Input: part model. Units: mm. Frame: model coordinates. A direction names the side the tool comes from. Coordinates: 2 decimals unless noted, no trailing zeros. Loops run counter-clockwise (first coordinate to the right, second up) from the corner with the lowest first, then second, coordinate; pieces in that order, holes last.
```python
from build123d import *

# Parameters (mm, degrees)
SKETCH1_W                                           = 68.2625
SKETCH1_H                                           = 190.5
BOSS_EXTRUDE1_DEPTH                                 = 20
CHAMFER1_SIZE                                       = 4
M8_TAPPED_HOLE1_D                                   = 6.8
F_8_0_8_DIAMETER_HOLE1_D                            = 8
CUT_EXTRUDE1_DEPTH                                  = 11
FILLET1_R                                           = 0.254
CBORE_FOR_M6_HEX_SOCKET_HEAD_CAP_SCREW1_D           = 6.6
CBORE_FOR_M6_HEX_SOCKET_HEAD_CAP_SCREW1_CBORE_D     = 11
CBORE_FOR_M6_HEX_SOCKET_HEAD_CAP_SCREW1_CBORE_DEPTH = 7
M6_TAPPED_HOLE1_D                                   = 5
M6_TAPPED_HOLE1_DEPTH                               = 27.9908
M6_TAPPED_HOLE1_TIP                                 = 1.502151548


with BuildPart() as part:
    # Sketch1 → Boss-Extrude1 (new body)
    with BuildSketch(Plane(origin=(0, 0, 0), x_dir=(1, 0, 0), z_dir=(0, 1, 0))):
        with Locations((-34.13125, 0)):
            Rectangle(SKETCH1_W, SKETCH1_H)
    extrude(amount=BOSS_EXTRUDE1_DEPTH)

    # Chamfer1
    chamfer1_edges = [part.edges().sort_by_distance(p)[0] for p in [
        (-34.13125, 20, -95.25),
    ]]
    chamfer(chamfer1_edges, length=CHAMFER1_SIZE)

    # M8 Tapped Hole1 (through all)
    with Locations(Plane(origin=(0, 20, 0), x_dir=(1, 0, 0), z_dir=(0, 1, 0))):
        with Locations((-59.85, -62.25), (-54.1, -32.25), (-19.1, -32.25), (-59.85, 37.75), (-54.1, 67.75), (-19.1, 67.75)):
            Hole(M8_TAPPED_HOLE1_D / 2)

    # Ø8.0 (8) Diameter Hole1 (through all)
    with Locations(Plane(origin=(0, 20, 0), x_dir=(1, 0, 0), z_dir=(0, 1, 0))):
        with Locations((-59.85, 20.0208), (-59.85, -79.9792)):
            Hole(F_8_0_8_DIAMETER_HOLE1_D / 2)

    # Sketch6 → Cut-Extrude1 (cut)
    with BuildSketch(Plane.XZ):
        with BuildLine():
            Line((-68.2625, 85.1242), (-54.85, 85.1242))
            ThreePointArc((-54.85, 85.1242), (-49.705, 79.9792), (-54.85, 74.8342))
            Line((-54.85, 74.8342), (-68.2625, 74.8342))
            ThreePointArc((-68.2625, 74.8342), (-73.4075, 79.9792), (-68.2625, 85.1242))
        make_face()
        with BuildLine():
            Line((-68.2625, -14.8758), (-54.85, -14.8758))
            ThreePointArc((-54.85, -14.8758), (-49.705, -20.0208), (-54.85, -25.1658))
            Line((-54.85, -25.1658), (-68.2625, -25.1658))
            ThreePointArc((-68.2625, -25.1658), (-73.4075, -20.0208), (-68.2625, -14.8758))
        make_face()
    extrude(amount=-CUT_EXTRUDE1_DEPTH, mode=Mode.SUBTRACT)

    # Fillet1
    fillet1_edges = [part.edges().sort_by_distance(p)[0] for p in [
        (-61.55625, 11, 85.1242),
        (-49.705, 11, 79.9792),
        (-61.55625, 11, 74.8342),
        (-61.55625, 11, -14.8758),
        (-49.705, 11, -20.0208),
        (-61.55625, 11, -25.1658),
    ]]
    fillet(fillet1_edges, radius=FILLET1_R)

    # CBORE for M6 Hex Socket Head Cap Screw1 (through all)
    with Locations(Plane(origin=(0, 0, 0), x_dir=(-1, 0, 0), z_dir=(0, -1, 0))):
        with Locations((9.849999954, 86.434800002), (39.849999954, 86.434800002), (39.849999954, -13.565199998), (9.849999954, -13.565199998)):
            CounterBoreHole(CBORE_FOR_M6_HEX_SOCKET_HEAD_CAP_SCREW1_D / 2, CBORE_FOR_M6_HEX_SOCKET_HEAD_CAP_SCREW1_CBORE_D / 2, CBORE_FOR_M6_HEX_SOCKET_HEAD_CAP_SCREW1_CBORE_DEPTH)

    # M6 Tapped Hole1
    with Locations(Plane(origin=(0, 0, 0), x_dir=(-1, 0, 0), z_dir=(0, -1, 0))):
        with Locations((42.35, 21.249999996), (42.35, 53.249999996)):
            Hole(M6_TAPPED_HOLE1_D / 2, depth=M6_TAPPED_HOLE1_DEPTH)
            with Locations((0, 0, -(M6_TAPPED_HOLE1_DEPTH + M6_TAPPED_HOLE1_TIP / 2))):  # 118° drill point
                Cone(0, M6_TAPPED_HOLE1_D / 2, M6_TAPPED_HOLE1_TIP, mode=Mode.SUBTRACT)


solid = part.part
```
Item 1: Mould query, pull axis X, two halves, no side actions, for faces 4 (the face through (-56.9, 11, 76.8)), 5 (the face through (-9, 3, 19)), 6 (the face through (-49.706, 5.298, -19.908)). Classes: +X half, -X half, draft (parallel to the pull), parting line (faces both ways), or undercut.
Result:
face 4: draft
face 5: undercut
face 6: -X half
Item 2: Section query D-D (y = 12.75). Count the separate pieces of the cut face and the enclosed holes in it, then the cut area to 3 significant figures.
Result:
separate pieces: 1
enclosed holes: 14
area: 12,500 mm2
Item 3: Section query B-B (z = 32.25). Output: boundary loops of the cut face in (x, y).
Result:
outline: (-68.26, 0) - (-57.5, 0) - (-57.5, 20) - (-68.26, 20) - close; (-50.7, 0) - (-22.5, 0) - (-22.5, 20) - (-50.7, 20) - close; (-15.7, 0) - (0, 0) - (0, 20) - (-15.7, 20) - close
Item 4: Contact query for flat-ended pins moving along their axis: P1, Ø5.5, axis at x = -19.1, z = -67.75, coming from the +Y side; P2, Ø5.5, axis at x = -7.5, z = -87, coming from the -Y side. Output: stop coordinate, or through.
Result:
P1: passes through
P2: stops at y = 7
Item 5: Section query A-A (x = -19.1). Output: boundary loops of the cut face in (y, z).
Result:
outline: (0, -95.25) - (16, -95.25) - (20, -91.25) - (20, -71.15) - (0, -71.15) - close; (0, -64.35) - (20, -64.35) - (20, 28.85) - (0, 28.85) - close; (0, 35.65) - (20, 35.65) - (20, 95.25) - (0, 95.25) - close
Item 6: Section query C-C (z = -53.25). Output: boundary loops of the cut face in (x, y).
Result:
outline: (-68.26, 0) - (-44.85, 0) - (-44.85, 20) - (-68.26, 20) - close; (-39.85, 0) - (0, 0) - (0, 20) - (-39.85, 20) - close
Item 7: Line query: L1, parallel to Z at x = -54, y = 13.5; L2, parallel to Z at x = -9.85, y = 13.25; L3, parallel to X at y = 4, z = -67.75. Output: solid intervals per line, ascending.
Result:
L1: z = -95.25 to -71.15, -64.35 to 28.85, 35.65 to 95.25
L2: z = -95.25 to -89.73, -83.13 to 10.27, 16.87 to 95.25
L3: x = -68.26 to -57.5, -50.7 to -22.5, -15.7 to 0
Item 8: Reachability of faces 1 (the face through (-62.99, 9.86, 63.55)), 2 (the face through (-61, 5, -25.166)), 3 (the face through (-43.4, 7, 13.5)) from +Z, -Z, +X, -X, +Y, -Y: full face, straight path, thin tool, end or side. Return the list, or none.
Result:
face 1: +Y, -Y
face 2: -X, -Y
face 3: -Y
